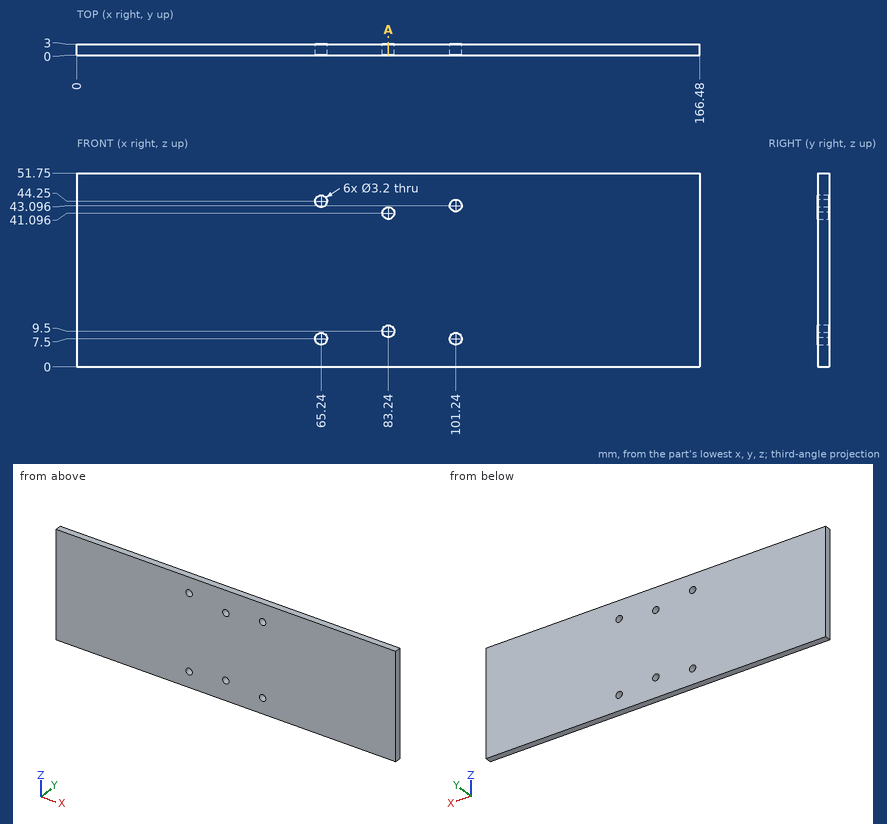
Source: three-view drawing plus pictorial views. Frame: mm from the lowest corner of the part. Give positions to 0.01 mm unless a question says otherwise; leave off trailing zeros. Write each loop counter-clockwise with the first axis right and the second up, starting at its lowest first coordinate (ties: lowest second). Pieces come first, ordered by that corner, then holes. Notation, with made-up numbers: (8, -13) - (37, -13) arc R20 cw to (37, 10) - close; hole circle Ø10 at (-5.75, 64.25). An arc over 180 degrees is marked (long way). Write item = value, one per line. Start each with the question number.
Q1. Material intervals for probe 1 along Z at (x, y) = (65.24, 1.15); probe 2 along Z at (x, y) = (83.24, 0.7); probe 3 along X at (y, z) = (2.15, 44.5), sorted ascending.
Q2. Pin query (flat end, axial travel): pin 1 Ø6 at (x, z) = (85.5, 27) entering from -Y. Return the tip coordinate at first contact, or that it passes through.
Q3. Cut plane A-A, the plane x = 83.24. Return loops of the section in (y, z), then the cut area to 3 significant figures.
Computed values:
q1.probe_1 = 0 to 5.9, 9.1 to 42.65, 45.85 to 51.75
q1.probe_2 = 0 to 7.9, 11.1 to 39.5, 42.7 to 51.75
q1.probe_3 = 0 to 63.66, 66.82 to 100.47, 102.01 to 166.48
q2.pin_1 = 0
q3.outline = (0, 0) - (3, 0) - (3, 7.9) - (0, 7.9) - close; (0, 11.1) - (3, 11.1) - (3, 39.5) - (0, 39.5) - close; (0, 42.7) - (3, 42.7) - (3, 51.75) - (0, 51.75) - close
q3.area = 136 mm²
